Source: CAD feature listing. Evaluate the final solid. Frame: model axes, mm. A direction names the side the tool comes from. Round coordinates to 2 decimals unless told otherwise and drop trailing zeros. Loops run counter-clockwise (first coordinate to the right, second up) from the corner with the lowest first, then second, coordinate; pieces in that order, holes last.
Item 1: Pull-direction query (X, two-part tool) for faces 1 (the flat face through (0, 35, -7)), 2 (the flat face through (-35, 0, -7)), 3 (the flat face through (32, 0, -7)); classes: released by +X, released by -X, zero draft, split by the parting line, or undercut.
Item 2: Access query for faces 4 (the flat face through (-32, 0, -7)), 5 (the flat face through (-34, 0, 535)). Directions: +Z, -Z, +X, -X, +Y, -Y. A direction counts if a zero-diameter tool reaches every point of the face in a straight line with its end or side. Return the directions, or none.
Item 3: Ray query, L1, parallel to Y at x = 2.5, z = -211; L2, parallel to X at y = 31, z = 146.5. Return the intervals inside material, ascending.
Item 4: Section query A-A on z = -399. Return loops of the section in (x, y), then the cut area to 3 significant figures.
Item 5: Section query B-B on y = 15. Return loops of the section in (x, z), then the cut area to 3 significant figures.
Autodesk Inventor part; units mm, degrees
ref_plane "Plano inicial" through (0, 0, -535) normal (0, 0, 1) x (1, 0, 0)
ref_plane "Plano final" through (0, 0, 535) normal (0, 0, 1) x (1, 0, 0)
ref_plane "Plano de trabajo4" through (2315, -29, -535) normal (0, 0, -1) x (-1, 0, 0)
ref_plane "Plano inicial" through (0, 0, -535) normal (0, 0, 1) x (1, 0, 0)
ref_plane "Plano final" through (0, 0, 535) normal (0, 0, 1) x (1, 0, 0)
sketch "Boceto" plane through (0, 0, 0) normal (0, 0, 1) x (1, 0, 0)
  line L0 (-35, -29) -> (-35, 29)
  line L1 (-29, 35) -> (29, 35)
  line L2 (35, 29) -> (35, -29)
  line L3 (29, -35) -> (-29, -35)
  arc A0 (-35, -29) -> (-29, -35) centre (-29, -29) ccw
  arc A1 (35, 29) -> (29, 35) centre (29, 29) ccw
  arc A2 (-29, 35) -> (-35, 29) centre (-29, 29) ccw
  arc A3 (29, -35) -> (35, -29) centre (29, -29) ccw
  arc A4 (-29, 32) -> (-32, 29) centre (-29, 29) ccw
  line L4 (-29, 32) -> (29, 32)
  arc A5 (32, 29) -> (29, 32) centre (29, 29) ccw
  line L5 (32, 29) -> (32, -29)
  arc A6 (29, -32) -> (32, -29) centre (29, -29) ccw
  line L6 (29, -32) -> (-29, -32)
  arc A7 (-32, -29) -> (-29, -32) centre (-29, -29) ccw
  line L7 (-32, -29) -> (-32, 29)
  line L8 (0, 50.7397) -> (0, -50.7397) construction
  line L9 (-50.7397, 0) -> (50.7397, 0) construction
  dimension "d7" = 6
  dimension "d9" = 70
  dimension "d11" = 70
  dimension "d12" = 3
  dimension "d15" = 35
  dimension "d16" = 35
extrude "Cuerpo" add sketch "Boceto" along normal up to surface (1070 mm away) from surface at -535
sketch "Sketch3" plane through (0, 0, 0) normal (0, 0, 1) x (1, 0, 0)
  line L0 (0, 0) -> (10, 0)
ref_plane "Work Plane3" through (0, 0, 0) normal (0, -1, 0) x (1, 0, 0)
sketch "Sketch4" plane through (0, 0, 0) normal (0, -1, 0) x (1, 0, 0)
  line L0 (-2, -535) -> (12, -535)
  line L1 (-2, 535) -> (12, 535)
  dimension "d18" = 1070
ref_plane "Plano de trabajo4" through (2315, -29, -535) normal (0, 0, -1) x (-1, 0, 0)
split "Dividir1" plane through (2315, -29, -535) removes the side toward (0, 0, -1)
ref_plane "Plano de trabajo5" through (0, -29, 535) normal (0, 0, 1) x (1, 0, 0)
split "Dividir2" plane through (0, -29, 535) removes the side toward (0, 0, 1)
equation "\"d7\" = G_IR"
equation "\"d9\" = G_W"
equation "\"d11\" = G_H"
equation "\"d12\" = G_T"
equation "\"d15\" = 0.5 * d9"
equation "\"d16\" = 0.5 * d11"
equation "\"d3\" = G_L"
equation "\"G_W\" = 70"
equation "\"G_H\" = 70"
equation "\"G_T\" = 3"
equation "\"G_IR\" = 6"
equation "\"G_L\" = d18"
equation "\"G_OFFSET_START\" = 535"
equation "\"G_OFFSET_END\" = 35"
equation "\"d13\" = -G_OFFSET_START"
equation "\"d14\" = G_OFFSET_END + B_L"
properties part number "ISO 10799-2 - 70x70x3 - 1070" material "Galvanizado catalogo 2"
Data:
1. face 1: zero draft
1. face 2: released by -X
1. face 3: undercut
2. face 4: +Z, -Z
2. face 5: +Z, +X, -X, +Y, -Y
3. L1: y = -35 to -32, 32 to 35
3. L2: x = -34.66 to -31.24, 31.24 to 34.66
4. outline: (-35, -29) arc R6 ccw to (-29, -35) - (29, -35) arc R6 ccw to (35, -29) - (35, 29) arc R6 ccw to (29, 35) - (-29, 35) arc R6 ccw to (-35, 29) - close; hole (-32, -29) arc R3 ccw to (-29, -32) - (29, -32) arc R3 ccw to (32, -29) - (32, 29) arc R3 ccw to (29, 32) - (-29, 32) arc R3 ccw to (-32, 29) - close
4. area: 781 mm2
5. outline: (-35, -535) - (-32, -535) - (-32, 535) - (-35, 535) - close; (32, -535) - (35, -535) - (35, 535) - (32, 535) - close
5. area: 6,420 mm2
